from build123d import *

# Parameters (mm, degrees)
SALIENTE_EXTRUIR1_DEPTH = 2.5
CROQUIS2_W              = 83
CROQUIS2_H              = 80
SALIENTE_EXTRUIR2_DEPTH = 65
CORTAR_EXTRUIR1_DEPTH   = 71
CROQUIS4_R              = 2.625
CORTAR_EXTRUIR2_DEPTH   = 68.5


with BuildPart() as part:
    # Croquis1 → Saliente-Extruir1 (new body)
    with BuildSketch(Plane(origin=(0, 0, 0), x_dir=(1, 0, 0), z_dir=(0, 1, 0))):
        Polygon((41.5, -85), (81.5, -85), (81.5, 85), (-81.5, 85), (-81.5, -85), (-41.5, -85), (-41.5, -55), (41.5, -55), align=None)
    extrude(amount=SALIENTE_EXTRUIR1_DEPTH)

    # Croquis2 → Saliente-Extruir2 (add)
    with BuildSketch(Plane(origin=(0, 2.5, 0), x_dir=(1, 0, 0), z_dir=(0, 1, 0))):
        with Locations((0, -15)):
            Rectangle(CROQUIS2_W, CROQUIS2_H)
    extrude(amount=SALIENTE_EXTRUIR2_DEPTH)

    # Croquis3 → Cortar-Extruir1 (cut, through all)
    with BuildSketch(Plane(origin=(0, 70, 0), x_dir=(1, 0, 0), z_dir=(0, 1, 0))):
        Polygon((-41.5, -15), (-41.5, -14.8), (41.5, -14.8), (41.5, -15.2), (-41.5, -15.2), align=None)
    extrude(amount=-CORTAR_EXTRUIR1_DEPTH, mode=Mode.SUBTRACT)

    # Croquis4 → Cortar-Extruir2 (cut, through all)
    with BuildSketch(Plane(origin=(0, 0, 0), x_dir=(1, 0, 0), z_dir=(0, 1, 0))):
        with Locations((-55.9, -64)):
            Circle(CROQUIS4_R)
        with Locations((55.9, -64)):
            Circle(CROQUIS4_R)
        with Locations((-55.9, 64)):
            Circle(CROQUIS4_R)
        with Locations((55.9, 64)):
            Circle(CROQUIS4_R)
    extrude(amount=CORTAR_EXTRUIR2_DEPTH, mode=Mode.SUBTRACT)


solid = part.part
Check sheet for the modelled part. Datum: model origin and axes. Units: mm. A direction names the side the tool comes from. Give positions to 0.01 mm unless a question says otherwise; leave off trailing zeros. Order: outer loops, then holes, each group sorted by start corner. A loop starts at its lowest first (then second) coordinate and runs counter-clockwise, first axis right, second up. Notation, with made-up numbers: (7, 16) - (49, 16) arc R21 cw to (49, 45) - close; hole circle Ø9 at (-18, -14). An arc over 180 degrees is marked (long way). Answer as CSV lines item,"result".
1. Mould release check, pull along X, two halves, no side actions. Record for faces 6 (the face through (-1, 2.5, -39)), 7 (the face through (41.5, 35, 35)), 8 (the face through (-58.522, 1.232, 63.885)): released by +X, released by -X, zero draft, split by the parting line, or undercut.
Result sheet:
face 6,"zero draft"
face 7,"released by +X"
face 8,"undercut"
2. Section check B-B (x = -55.9). Record the boundary of the cut face in (y, z) (3 decimals).
Result sheet:
outline,"(0, -85) - (2.5, -85) - (2.5, -66.625) - (0, -66.625) - close; (0, -61.375) - (2.5, -61.375) - (2.5, 61.375) - (0, 61.375) - close; (0, 66.625) - (2.5, 66.625) - (2.5, 85) - (0, 85) - close"
3. Section check C-C (z = 64). Record the boundary of the cut face in (x, y) (3 decimals), then the cut area to 3 significant figures.
Result sheet:
outline,"(-81.5, 0) - (-58.525, 0) - (-58.525, 2.5) - (-81.5, 2.5) - close; (-53.275, 0) - (-41.5, 0) - (-41.5, 2.5) - (-53.275, 2.5) - close; (41.5, 0) - (53.275, 0) - (53.275, 2.5) - (41.5, 2.5) - close; (58.525, 0) - (81.5, 0) - (81.5, 2.5) - (58.525, 2.5) - close"
area,"174 mm²"
4. Section check A-A (y = 50). Record the boundary of the cut face in (x, z).
Result sheet:
outline,"(-41.5, -25) - (41.5, -25) - (41.5, 14.8) - (-41.5, 14.8) - close; (-41.5, 15.2) - (41.5, 15.2) - (41.5, 55) - (-41.5, 55) - close"
5. Go/stop test with flat-tipped pins: P1, Ø20, axis at y = 19.5, z = 41, coming from the +X side; P2, Ø3, axis at x = -55.9, z = 64, coming from the -Y side; P3, Ø8, axis at x = 17.5, y = 36.5, coming from the +Z side; P4, Ø2, axis at x = 9, y = 38, coming from the -Z side. Record where each tip stops, or that it passes through.
Result sheet:
P1,"x = 41.5"
P2,"through"
P3,"z = 55"
P4,"z = -25"
6. Tool access check on faces 1 (the face through (-1, 35, -25)), 2 (the face through (53.278, 1.232, -64.115)), 3 (the face through (-41.5, 35, 35)), 4 (the face through (-1, 0, -1)), 5 (the face through (41.5, 35, -5)). Record the directions out of +Z, -Z, +X, -X, +Y, -Y that give a thin tool (end or side, any length) a straight path to the whole face; none if there is none.
Result sheet:
face 1,"-Z, +X, -X, +Y"
face 2,"+Y, -Y"
face 3,"+Z, -Z, -X, +Y"
face 4,"+Z, -Z, +X, -X, -Y"
face 5,"+Z, -Z, +X, +Y"
7. Scan lines: probe 1 along Z at (x, y) = (-55.9, 0.95) (3 decimals); probe 2 along Z at (x, y) = (25.5, 49); probe 3 along X at (y, z) = (1.8, 64) (3 decimals). Record each from-to range of solid material in increasing order. Write a range as from..to.
Result sheet:
probe 1,"-85..-66.625, -61.375..61.375, 66.625..85"
probe 2,"-25..14.8, 15.2..55"
probe 3,"-81.5..-58.525, -53.275..-41.5, 41.5..53.275, 58.525..81.5"
8. Section check D-D (x = -17). Record the boundary of the cut face in (y, z), then the cut area to 3 significant figures.
Result sheet:
outline,"(0, -85) - (2.5, -85) - (2.5, -25) - (67.5, -25) - (67.5, 14.8) - (0, 14.8) - close; (0, 15.2) - (67.5, 15.2) - (67.5, 55) - (0, 55) - close"
area,"5,520 mm²"
